from build123d import *

# Parameters (mm, degrees)
SKETCH1_W               = 57.15
SKETCH1_H               = 25.4
BOSS_EXTRUDE1_DEPTH     = 63.5
F_1_4_20_TAPPED_HOLE1_D = 5.1054
CUT_EXTRUDE1_DEPTH      = 75.121121315


with BuildPart() as part:
    # Sketch1 → Boss-Extrude1 (new body)
    with BuildSketch(Plane.XY):
        Rectangle(SKETCH1_W, SKETCH1_H)
    extrude(amount=BOSS_EXTRUDE1_DEPTH)

    # 1/4-20 Tapped Hole1 (through all)
    with Locations(Plane(origin=(28.575, 0, 0), x_dir=(0, 0, -1), z_dir=(1, 0, 0))):
        with Locations((-34.925, 0), (-9.525, 0)):
            Hole(F_1_4_20_TAPPED_HOLE1_D / 2)

    # Sketch5 → Cut-Extrude1 (cut, through all)
    with BuildSketch(Plane(origin=(0, 12.7, 0), x_dir=(1, 0, 0), z_dir=(0, 1, 0))):
        Polygon((-23.8252, -63.5), (0, -39.6748), (23.8252, -63.5), align=None)
    extrude(amount=-CUT_EXTRUDE1_DEPTH, mode=Mode.SUBTRACT)


solid = part.part
Geometry check sheet. Reference: the model listing, model coordinates, mm. A direction names the side the tool comes from. Give positions to 0.01 mm unless a question says otherwise; leave off trailing zeros. Order: outer loops, then holes, each group sorted by start corner. A loop starts at its lowest first (then second) coordinate and runs counter-clockwise, first axis right, second up.
1. Draft check along Z on faces 3 (the face through (-0.4, 1.725, 7.644)), 4 (the face through (26, 0, 63.5)), 5 (the face through (0, -12.7, 24)). Enter one of: pulls with the +Z half, pulls with the -Z half, needs draft (parallel to the pull), parting line crosses it, or undercut.
Completed:
face 3: undercut
face 4: pulls with the +Z half
face 5: needs draft
2. Scan lines: line 1 (Z direction, x = -5.5, y = 1.5); line 2 (Z direction, x = -17.5, y = 1); line 3 (X direction, y = 4.5, z = 54.5) (3 decimals). Record each from-to range of solid material in increasing order.
Completed:
line 1: z = 0 to 7.46, 11.59 to 32.86, 36.99 to 45.17
line 2: z = 0 to 7.18, 11.87 to 32.58, 37.27 to 57.17
line 3: x = -28.575 to -14.825, 14.825 to 28.575
3. Sectioned sample at A-A (y = 0). Record the boundary of the cut face in (x, z) (3 decimals).
Completed:
outline: (-28.575, 0) - (28.575, 0) - (28.575, 6.972) - (-28.575, 6.972) - close; (-28.575, 12.078) - (28.575, 12.078) - (28.575, 32.372) - (-28.575, 32.372) - close; (-28.575, 37.478) - (28.575, 37.478) - (28.575, 63.5) - (23.825, 63.5) - (0, 39.675) - (-23.825, 63.5) - (-28.575, 63.5) - close
4. Sectioned sample at C-C (y = -6). Record the boundary of the cut face in (x, z) (3 decimals), then the cut area to 3 significant figures.
Completed:
outline: (-28.575, 0) - (28.575, 0) - (28.575, 63.5) - (23.825, 63.5) - (0, 39.675) - (-23.825, 63.5) - (-28.575, 63.5) - close
area: 3,060 mm2
5. Sectioned sample at B-B (z = 49). Record the boundary of the cut face in (x, y) (3 decimals), then the cut area to 3 significant figures.
Completed:
outline: (-28.575, -12.7) - (-9.325, -12.7) - (-9.325, 12.7) - (-28.575, 12.7) - close; (9.325, -12.7) - (28.575, -12.7) - (28.575, 12.7) - (9.325, 12.7) - close
area: 978 mm2
6. Depth check by flat-ended pin: pin 1 (8 mm diameter, centred on x = -17, y = 9, fed in from +Z). Enter the tip coordinate at first touch or a pass-through.
Completed:
pin 1: stops at z = 60.67
7. Access from +Z, -Z, +X, -X, +Y, -Y to the whole of each face (thin tool, end or side, straight path). Record for faces 1 (the face through (-26, 0, 63.5)), 2 (the face through (11.746, 0.178, 51.421)).
Completed:
face 1: +Z, +X, -X, +Y, -Y
face 2: +Z, +Y, -Y
8. Sectioned sample at D-D (x = -18). Record the boundary of the cut face in (y, z) (3 decimals).
Completed:
outline: (-12.7, 0) - (12.7, 0) - (12.7, 57.675) - (-12.7, 57.675) - close; hole circle Ø5.105 at (0, 9.525); hole circle Ø5.105 at (0, 34.925)
